Autodesk Inventor part; units mm, degrees
ref_plane "YZ Plane" through (0, 0, 0) normal (1, 0, 0) x (0, 1, 0)
ref_plane "XZ Plane" through (0, 0, 0) normal (0, 1, 0) x (-1, 0, 0)
ref_plane "XY Plane" through (0, 0, 0) normal (0, 0, 1) x (1, 0, 0)
sketch "Sketch1" plane through (0, 0, 0) normal (1, 0, 0) x (0, 1, 0)
  line L0 (-58, -40) -> (-58, 50)
  line L1 (0, 0) -> (-57.3223, 54.5531) construction
  circle A0 centre (0, 0) radius 47 construction
  circle A1 centre (0, 0) radius 10
  line L2 (-11, -52) -> (14.1774, -52)
  line L3 (-58, 0) -> (-58, -40)
  line L4 (0, 0) -> (0, -52) construction
  line L5 (-58, -40) -> (-23, -52.739)
  circle A2 centre (0, 0) radius 50 construction
  arc A3 (22.2788, -50.2857) -> (0, 55) centre (0, 0) ccw
  line L6 (-43.4633, 41.3636) -> (-48.6337, 35.9307)
  arc A4 (-53, 55) -> (-58, 50) centre (-53, 50) ccw
  line L7 (-11, 54) -> (-11, 50)
  line L8 (-12, 49) -> (-22, 49)
  line L9 (-23, 50) -> (-23, 54)
  line L10 (-53, 55) -> (-24, 55)
  line L11 (-10, 55) -> (0, 55)
  arc A5 (-23, 54) -> (-24, 55) centre (-24, 54) ccw
  arc A6 (-10, 55) -> (-11, 54) centre (-10, 54) ccw
  arc A7 (-12, 49) -> (-11, 50) centre (-12, 50) ccw
  arc A8 (-23, 50) -> (-22, 49) centre (-22, 50) ccw
  arc A9 (14.1774, -52) -> (22.2788, -50.2857) centre (14.1774, -32) ccw
  line L12 (-23, -49.5) -> (-23, -52.739)
  line L13 (-11, -52) -> (-11, -49.5)
  line L14 (-11.5, -49) -> (-22.5, -49)
  arc A10 (-11, -49.5) -> (-11.5, -49) centre (-11.5, -49.5) ccw
  arc A11 (-22.5, -49) -> (-23, -49.5) centre (-22.5, -49.5) ccw
  line L15 (0, -52) -> (-10, -52)
  point P0 (-28.9755, 27.5757)
  point P1 (-57.7919, 55)
  point P2 (-58, 55)
  point P3 (-25.2108, 39.6663)
  point P4 (17.9165, -52)
  point P5 (-23, 55)
  point P6 (-11, 52)
  dimension "d4" = 94
  dimension "d8" = 60
  dimension "d9" = 20
  dimension "d13" = 52
  dimension "d20" = 100
  dimension "d31" = 55
  dimension "d34" = 58
  dimension "d52" = 5
  dimension "d54" = 47
  dimension "d56" = 1
  dimension "d59" = 20
  dimension "d60" = 12
  dimension "d61" = 6
  dimension "d65" = 0.5
  dimension "d71" = 95
  dimension "d74" = 110
  dimension "d75" = 12
  dimension "d76" = 3
extrude "Extrusion4" add sketch "Sketch1" along normal blind 1.5
fillet "Fillet1" radius 5 1 edges at (0.75, -58, -40)
fillet "Fillet2" radius 1.5 2 edges at (0.75, -23, -52.739) (0.75, -11, -52)
properties part number "OuterFlange27130914"
Design review of the part built by this model. Coordinates are the model's own, in mm. Coordinates: 2 decimals unless noted, no trailing zeros. Order: outer loops, then holes, each group sorted by start corner. A loop starts at its lowest first (then second) coordinate and runs counter-clockwise, first axis right, second up.
1) Mouldability with a two-part tool opening along Z and no side actions: class faces 1 (the cylindrical face through (0.74, -2.17, 9.76)), 2 (the cylindrical face through (0.74, 53.58, 12.41)), 3 (the cylindrical face through (0.76, -57.12, -39.33)) as +Z half, -Z half, draft (parallel to the pull), parting line (faces both ways), or undercut.
2) Take a section at C-C, the plane y = -42.5. Give the boundary of the cut face in (x, z).
3) Take a section at B-B, the plane y = 8. Give the boundary of the cut face in (x, z).
4) Take a section at A-A, the plane z = 0. Give the boundary of the cut face in (x, y).
5) Take a section at D-D, the plane z = -14.5. Give the boundary of the cut face in (x, y), and give its area (3 significant figures).
6) Clearance check with flat-ended pins moving along their axes: pin 1 (0.5 mm diameter, centred on x = 1, z = -50, fed in from +Y); pin 2 (0.8 mm diameter, centred on x = 0.5, y = -18, fed in from +Z); pin 3 (18 mm diameter, centred on y = 0, z = 0, fed in from -X); pin 4 (0.8 mm diameter, centred on x = 1, z = 52, fed in from -Y). State where each tip first meets the part, or that it passes through.
7) Wall thickness on line 1 along Z through (x, y) = (0.6, 0); line 2 along Y through (x, z) = (1.35, 7); line 3 along Z through (x, y) = (0.9, -15.5): over which ranges is each line inside the solid? List them lowest first.
Returned:
1. face 1: undercut
1. face 2: parting line
1. face 3: -Z half
2. outline: (0, -45.64) - (1.5, -45.64) - (1.5, 55) - (0, 55) - close
3. outline: (0, -52) - (1.5, -52) - (1.5, -6) - (0, -6) - close; (0, 6) - (1.5, 6) - (1.5, 54.42) - (0, 54.42) - close
4. outline: (0, -58) - (1.5, -58) - (1.5, -10) - (0, -10) - close; (0, 10) - (1.5, 10) - (1.5, 55) - (0, 55) - close
5. outline: (0, -58) - (1.5, -58) - (1.5, 53.05) - (0, 53.05) - close
5. area: 167 mm2
6. pin 1: stops at y = 23.45
6. pin 2: stops at z = 49
6. pin 3: passes through
6. pin 4: stops at y = -57.74
7. line 1: z = -52 to -10, 10 to 55
7. line 2: y = -58 to -7.14, 7.14 to 54.55
7. line 3: z = -49 to 49
